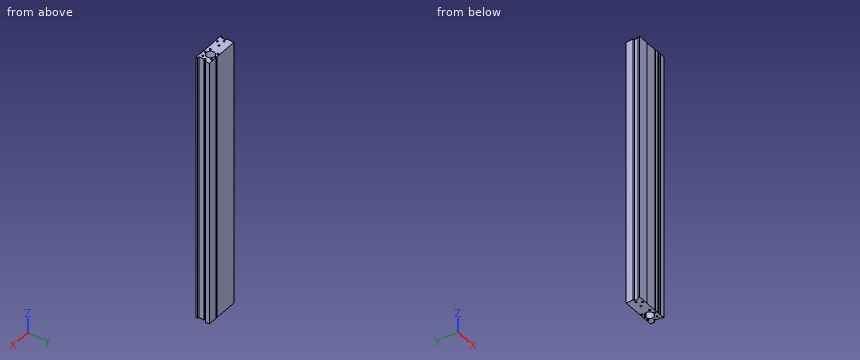
```python
from build123d import *

# Parameters (mm, degrees)
BASE_DEPTH                = 325
BASE_DEPTH_BACK           = 325
BASE_SKETCH_W             = 78
BASE_SKETCH_H             = 31.5
BASE_SKETCH_R             = 10
BASE_GROOVE_DEPTH         = 331.168896173
BASE_GROOVE_DEPTH_BACK    = 331.168896173
SEAL_GROOVE_DEPTH         = 331.168896173
SEAL_GROOVE_DEPTH_BACK    = 331.168896173
HOLES_DEPTH               = 331.168896173
HOLES_DEPTH_BACK          = 331.168896173
HOLES_SKETCH_R            = 2
SWITCH_GROOVE1_DEPTH      = 331.168896173
SWITCH_GROOVE1_DEPTH_BACK = 331.168896173
SIDE_GROOVE1_DEPTH        = 331.168896173
SIDE_GROOVE1_DEPTH_BACK   = 331.168896173
SIDE_GROOVE2_DEPTH        = 331.168896173
SIDE_GROOVE2_DEPTH_BACK   = 331.168896173


with BuildPart() as part:
    # Base_Sketch → Base (new, two sides: drawn at the far end of the back side and taken through both)
    with BuildSketch(Plane.XY.offset(-BASE_DEPTH_BACK)):
        with Locations((-16.5, -1.75)):
            Rectangle(BASE_SKETCH_W, BASE_SKETCH_H)
        Circle(BASE_SKETCH_R, mode=Mode.SUBTRACT)
    extrude(amount=BASE_DEPTH + BASE_DEPTH_BACK)

    # Base_Groove_Sketch → Base_Groove (cut, two sides: drawn at the far end of the back side and taken through both)
    with BuildSketch(Plane.XY.offset(-BASE_GROOVE_DEPTH_BACK)):
        Polygon((12, -17.5), (11.133974596, -17), (5.366025404, -17), (4.5, -17.5), align=None)
        Polygon((-4.5, -17.5), (-5.366025404, -17), (-30.633974596, -17), (-31.5, -17.5), align=None)
    extrude(amount=BASE_GROOVE_DEPTH + BASE_GROOVE_DEPTH_BACK, mode=Mode.SUBTRACT)

    # Seal_Groove_Sketch → Seal_Groove (cut, two sides: drawn at the far end of the back side and taken through both)
    with BuildSketch(Plane.XY.offset(-SEAL_GROOVE_DEPTH_BACK)):
        with BuildLine():
            Line((-1.45, 14), (-1.45, 9.89431655))
            ThreePointArc((-1.45, 9.89431655), (0, 10), (1.45, 9.89431655))
            Line((1.45, 9.89431655), (1.45, 14))
            Line((1.45, 14), (-1.45, 14))
        make_face()
    extrude(amount=SEAL_GROOVE_DEPTH + SEAL_GROOVE_DEPTH_BACK, mode=Mode.SUBTRACT)

    # Holes_Sketch → Holes (cut, two sides: drawn at the far end of the back side and taken through both)
    with BuildSketch(Plane.XY.offset(-HOLES_DEPTH_BACK)):
        with Locations((12, -9.5)):
            Circle(HOLES_SKETCH_R)
        with Locations((-12, -9.5)):
            Circle(HOLES_SKETCH_R)
        with Locations((10, 10.5)):
            Circle(HOLES_SKETCH_R)
        with Locations(Location((-10, 10.5, 0), (0, 0, 180))):
            Circle(HOLES_SKETCH_R)
        with Locations((0, -13)):
            Circle(HOLES_SKETCH_R)
        with Locations((-31, -3)):
            Circle(HOLES_SKETCH_R)
        with Locations((-47, -3)):
            Circle(HOLES_SKETCH_R)
        with Locations((-39, -13)):
            Circle(HOLES_SKETCH_R)
    extrude(amount=HOLES_DEPTH + HOLES_DEPTH_BACK, mode=Mode.SUBTRACT)

    # Switch_Groove1_Sketch (on Front Plane) → Switch_Groove1 (cut, two sides: drawn at the far end of the back side and taken through both)
    with BuildSketch(Plane.XY.offset(-SWITCH_GROOVE1_DEPTH_BACK)):
        with BuildLine():
            Line((22.5, 1.5), (18.469693846, 1.5))
            ThreePointArc((18.469693846, 1.5), (14.9, 0), (18.469693846, -1.5))
            Line((18.469693846, -1.5), (22.5, -1.5))
            Line((22.5, -1.5), (22.5, 1.5))
        make_face()
    extrude(amount=SWITCH_GROOVE1_DEPTH + SWITCH_GROOVE1_DEPTH_BACK, mode=Mode.SUBTRACT)

    # Side_Groove1_Sketch → Side_Groove1 (cut, two sides: drawn at the far end of the back side and taken through both)
    with BuildSketch(Plane.XY.offset(-SIDE_GROOVE1_DEPTH_BACK)):
        Polygon((-55.5, -14.5), (-52, -13.691961331), (-52, -3.308038669), (-55.5, -2.5), align=None)
    extrude(amount=SIDE_GROOVE1_DEPTH + SIDE_GROOVE1_DEPTH_BACK, mode=Mode.SUBTRACT)

    # Side_Groove2_Sketch → Side_Groove2 (cut, two sides: drawn at the far end of the back side and taken through both)
    with BuildSketch(Plane.XY.offset(-SIDE_GROOVE2_DEPTH_BACK)):
        Polygon((22.5, 4.5), (19, 3.691961331), (19, -13.691961331), (22.5, -14.5), align=None)
    extrude(amount=SIDE_GROOVE2_DEPTH + SIDE_GROOVE2_DEPTH_BACK, mode=Mode.SUBTRACT)


solid = part.part
```
Geometry check sheet. Reference: the model listing, model coordinates, mm. Round coordinates to 2 decimals unless told otherwise and drop trailing zeros. Use a Markdown table: item, result.
(1) Go/stop test with flat-tipped pins: P1, Ø4, axis at y = -10.5, z = 201, coming from the -X side; P2, Ø10, axis at y = -7.5, z = -3, coming from the +X side; P3, Ø6.5, axis at x = 9.5, z = -66, coming from the -Y side; P4, Ø1, axis at x = -9, z = -113, coming from the -Y side. Record where each tip stops, or that it passes through.
Calculated:
| item | result |
|---|---|
| P1 | x = -52 |
| P2 | x = 19 |
| P3 | y = -17.5 |
| P4 | y = -17 |
(2) Sectioned sample at A-A (z = -107). Give the number of separate pieces and of enclosed holes in the cut face, then the cut area to 3 significant figures.
Calculated:
| item | result |
|---|---|
| separate pieces | 1 |
| enclosed holes | 8 |
| area | 1,900 mm² |
(3) Scan lines: probe 1 along X at (y, z) = (-12.5, -78); probe 2 along Y at (x, z) = (0, 147); probe 3 along Y at (x, z) = (-47, 92). Record each from-to range of solid material in increasing order.
Calculated:
| item | result |
|---|---|
| probe 1 | -52 to -40.94, -37.06 to -1.94, 1.94 to 19 |
| probe 2 | -17.5 to -15, -11 to -10 |
| probe 3 | -17.5 to -5, -1 to 14 |
